The model under review builds one solid part; all positions refer to its coordinate system, in mm. A direction names the side the tool comes from. Coordinates: 2 decimals unless noted, no trailing zeros. Order: outer loops, then holes, each group sorted by start corner. A loop starts at its lowest first (then second) coordinate and runs counter-clockwise, first axis right, second up. Notation, with made-up numbers: (67, -30.75) -> (96, -30.75) arc R27 ccw to (96, -3.75) -> close; hole circle Ø9 at (-26, 21). An arc over 180 degrees is marked (long way). Use one line per item in the form item = value. Start each with the question number.
(1) Take a section at A-A (x = 0). State the section outline as (y, z) points.
(2) Mouldability with a two-part tool opening along X and no side actions: class faces 1 (the cylindrical face through (-13.887, -31.552, -10.648)), 2 (the flat face through (-20, 20, -9)), 3 (the flat face through (17.5, 27, -20)) as +X half, -X half, draft (parallel to the pull), parting line (faces both ways), or undercut.
(3) Take a section at D-D (y = 4). State the section outline as (x, z) points.
(4) Take a section at C-C (z = -14). State the section outline as (x, y) points.
(5) Insertion check: pin 1 Ø3 at (y, z) = (-5, -7.5) entering from -X; pin 2 Ø6 at (y, z) = (-50.5, -18) entering from +X; pin 3 Ø6.5 at (x, z) = (5.5, -16.5) entering from +Y. Each pin has a flat end and moves straight along its axis. Give the tip position at first contact, or say it passes through.
(6) Wall thickness on line 1 along Z through (x, y) = (-8.5, 12.5); line 2 along X through (y, z) = (6, 0); line 3 along X through (y, z) = (28, 23): over which ranges is each line inside the solid? List them lowest first.
(7) Take a section at B-B (z = 0). State the section outline as (x, y) points, then the cut area to 3 significant figures.
(8) For faces 4 (the flat face through (17.5, 27, 19)), 5 (the flat face through (24, 32, 20)), 6 (the flat face through (20, 20, -9)), list the 3-axis set-ups (+Z, -Z, +X, -X, +Y, -Y) from which the entire face can be reached by the end or side of a thin tool; tool diameter is ignored.
```python
from build123d import *

# Parameters (mm, degrees)
F0_R     = 17.5
F0_R_2   = 10
F1_DEPTH = 64
F2_W     = 60
F2_H     = 60
F2_R     = 17.5
F2_R_2   = 10
F3_DEPTH = 32
F4_W     = 35
F4_H     = 10
F5_DEPTH = 60.001
F6_W     = 20
F6_H     = 18
F7_DEPTH = 60.001


with BuildPart() as f1:
    # F0 (on Front) → F1 (new body)
    with BuildSketch(Plane.XZ):
        Circle(F0_R)
        Circle(F0_R_2, mode=Mode.SUBTRACT)
    extrude(amount=F1_DEPTH)

    # F2 (on face) → F3 (join)
    with BuildSketch(Plane(origin=(0, 0, 0), x_dir=(-1, 0, 0), z_dir=(0, 1, 0))):
        Rectangle(F2_W, F2_H)
        Circle(F2_R, mode=Mode.SUBTRACT)
        Circle(F2_R)
        Circle(F2_R_2, mode=Mode.SUBTRACT)
    extrude(amount=F3_DEPTH)

    # F4 (on face) → F5 (cut, through all)
    with BuildSketch(Plane(origin=(0, 0, -30), x_dir=(1, 0, 0), z_dir=(0, 0, -1))):
        with Locations((0, -27)):
            Rectangle(F4_W, F4_H)
    extrude(amount=-F5_DEPTH, mode=Mode.SUBTRACT)

    # F6 (on face) → F7 (cut, through all)
    with BuildSketch(Plane(origin=(-30, 0, 0), x_dir=(0, -1, 0), z_dir=(-1, 0, 0))):
        with Locations((-22, 0)):
            Rectangle(F6_W, F6_H)
    extrude(amount=-F7_DEPTH, mode=Mode.SUBTRACT)


solid = f1.part
```
Findings:
q1.outline = (-64, -17.5) -> (0, -17.5) -> (0, -30) -> (22, -30) -> (22, -10) -> (-64, -10) -> close; (-64, 10) -> (22, 10) -> (22, 30) -> (0, 30) -> (0, 17.5) -> (-64, 17.5) -> close
q2.face_1 = parting line
q2.face_2 = draft
q2.face_3 = undercut
q3.outline = (-30, -30) -> (30, -30) -> (30, 30) -> (-30, 30) -> close; hole circle Ø20 at (0, 0)
q4.outline = (-30, 0) -> (-10.5, 0) -> (-10.5, -64) -> (10.5, -64) -> (10.5, 0) -> (30, 0) -> (30, 32) -> (17.5, 32) -> (17.5, 22) -> (-17.5, 22) -> (-17.5, 32) -> (-30, 32) -> close
q5.pin_1 = -16.44
q5.pin_2 = 9.01
q5.pin_3 = 22
q6.line_1 = -30 to -9, 9 to 30
q6.line_2 = -30 to -10, 10 to 30
q6.line_3 = -30 to -17.5, 17.5 to 30
q7.outline = (-30, 0) -> (-17.5, 0) -> (-17.5, -64) -> (-10, -64) -> (-10, 12) -> (-30, 12) -> close; (10, -64) -> (17.5, -64) -> (17.5, 0) -> (30, 0) -> (30, 12) -> (10, 12) -> close
q7.area = 1,440 mm²
q8.face_4 = +Z, -Z, +Y
q8.face_5 = +Z, -Z, +X, -X, +Y
q8.face_6 = +X, -X, +Y
